```python
from build123d import *

# Parameters (mm, degrees)
F0_W     = 38.1
F0_H     = 88.9
F1_DEPTH = 254
F3_DEPTH = 38.101
F5_D     = 6.35
F6_R     = 5.08
F8_D     = 6.35
F8_DEPTH = 25.4
F8_TIP   = 1.9077324654


with BuildPart() as f1:
    # F0 (on Top) → F1 (new body, symmetric)
    with BuildSketch(Plane.XY):
        Rectangle(F0_W, F0_H)
    extrude(amount=F1_DEPTH, both=True)

    # F2 (on face) → F3 (cut, through all)
    with BuildSketch(Plane.YZ.offset(19.05)):
        Polygon((-44.45, 254), (-44.45, 212.54524919), (44.45, 254), align=None)
        Polygon((-6.8792365313, -236.4804652718), (-44.45, -254), (44.45, -254), (44.45, -212.54524919), align=None)
        Polygon((-44.45, -155.9097030042), (-44.45, -254), (-6.8792365313, -236.4804652718), align=None)
    extrude(amount=-F3_DEPTH, mode=Mode.SUBTRACT)

    # F5 (through all)
    with Locations(Plane.YZ.offset(19.05)):
        with Locations((-10.6952783611, -168.1954169468), (5.4064774113, -202.7257436328)):
            Hole(F5_D / 2)

    # F6
    f6_edges = [f1.edges().sort_by_distance(p)[0] for p in [
        (19.05, -44.45, 28.317773),
        (-19.05, -44.45, 28.317773),
        (19.05, 44.45, 20.727375),
        (-19.05, 44.45, 20.727375),
    ]]
    fillet(f6_edges, radius=F6_R)

    # F8
    with Locations(Plane(origin=(0, -89.3485989014, 191.6086886819), x_dir=(1, 0, 0), z_dir=(0, -0.4226182617, 0.906307787))):
        with Locations((0, 113.0401226202), (0, 74.9401226202)):
            Hole(F8_D / 2, depth=F8_DEPTH)
            with Locations((0, 0, -(F8_DEPTH + F8_TIP / 2))):  # 118° drill point
                Cone(0, F8_D / 2, F8_TIP, mode=Mode.SUBTRACT)


solid = f1.part
```
Input: part model. Units: mm. Frame: model coordinates. Give positions to 0.01 mm unless a question says otherwise; leave off trailing zeros. Write each loop counter-clockwise with the first axis right and the second up, starting at its lowest first coordinate (ties: lowest second). Pieces come first, ordered by that corner, then holes. Notation, with made-up numbers: (52, 73.25) - (58, 73.25) arc R15 ccw to (58, 82.25) - close; hole circle Ø1 at (-24.5, 57). An arc over 180 degrees is marked (long way). Write item = value, one per line. Start each with the question number.
1. Section query A-A, the plane x = 9.5. Output: boundary loops of the cut face in (y, z) (3 decimals).
2. Section query C-C, the plane y = -33.5. Output: boundary loops of the cut face in (x, z).
3. Section query B-B, the plane z = -160. Output: boundary loops of the cut face in (x, y), then the cut area to 3 significant figures.
4. Mould query, pull axis X, two halves, no side actions, for faces 1 (the flat face through (-19.05, -1, 11)), 2 (the flat face through (0, 44.45, 24)), 3 (the cylindrical face through (0.413, 21.396, 229.041)). Classes: released by +X, released by -X, zero draft, split by the parting line, or undercut.
5. Ray query, L1, parallel to Z at x = 6, y = 5; L2, parallel to Z at x = 5.5, y = 6.5 (3 decimals); L3, parallel to Y at x = 5.5, z = -167.5. Return the intervals inside material, ascending.
6. Section query D-D, the plane y = 34. Output: boundary loops of the cut face in (x, z).
7. First-contact query: pin 1 Ø12 at (x, y) = (-6.5, 27.5) entering from -Z; pin 2 Ø1 at (x, y) = (-12.5, 2.5) entering from +Z; pin 3 Ø4 at (x, y) = (-3, 6.5) entering from +Z. Flat tips, straight axial feed; report the tip coordinate or a pass-through.
Check sheet entries:
q1.outline = (-44.45, -155.91) - (-6.879, -236.48) - (44.45, -212.545) - (44.45, 254) - (-44.45, 212.545) - close; hole circle Ø6.35 at (-10.695, -168.195); hole circle Ø6.35 at (5.406, -202.726)
q2.outline = (-19.05, -179.39) - (19.05, -179.39) - (19.05, 217.65) - (-19.05, 217.65) - close
q3.outline = (-19.05, -39.37) arc R5.08 ccw to (-17.94, -42.54) - (17.94, -42.54) arc R5.08 ccw to (19.05, -39.37) - (19.05, 39.37) arc R5.08 ccw to (13.97, 44.45) - (-13.97, 44.45) arc R5.08 ccw to (-19.05, 39.37) - close
q3.area = 3,300 mm2
q4.face_1 = released by -X
q4.face_2 = zero draft
q4.face_3 = undercut
q5.L1 = -230.94 to -205.87, -199.58 to 235.6
q5.L2 = -230.242 to -205.706, -199.745 to 236.304
q5.L3 = -39.05 to -13.79, -7.6 to 44.45
q6.outline = (-19.05, -217.42) - (19.05, -217.42) - (19.05, 249.13) - (-19.05, 249.13) - close
q7.pin_1 = -223.25
q7.pin_2 = 234.67
q7.pin_3 = 237.24
